Work out the finished part from the listing and answer in its coordinate system (mm). Give positions to 0.01 mm unless a question says otherwise; leave off trailing zeros. Write each loop counter-clockwise with the first axis right and the second up, starting at its lowest first coordinate (ties: lowest second). Pieces come first, ordered by that corner, then holes. Notation, with made-up numbers: (-3.75, 69) -> (50.25, 69) arc R34 ccw to (50.25, 102) -> close; hole circle Ø9 at (86.5, 26). An arc over 180 degrees is marked (long way). Use a Markdown table: item, result. Add a question column.
Q1. Section C-C, the plane x = -95.25 is taken. Give the vertices of the cut face in (y, z).
Q2. Section B-B, the plane y = 19.05 is taken. Give the vertices of the cut face in (x, z) (3 decimals), plus the area to 3 significant figures.
Q3. Each of these flat-tipped pins is pushed along its axis until it touches: pin 1 Ø3.5 at (x, z) = (82.55, 6.35) entering from -Y; pin 2 Ø9 at (x, y) = (84.78, 19.05) entering from +Z; pin 3 Ø3 at (x, z) = (0, 6.35) entering from -Y. Where does it stop, or does it pass through?
Q4. Consider line 1 (X direction, y = -63.5, z = 5.5); line 2 (Y direction, x = -95.25, z = 6.75); line 3 (X direction, y = -61.5, z = 2.5). Determine where each line is inside the solid, lowest interval first.
Q5. Section A-A, the plane y = -63.5 is taken. Give the vertices of the cut face in (x, z).
Q6. Section D-D, the plane y = -5 is taken. Give the vertices of the cut face in (x, z).
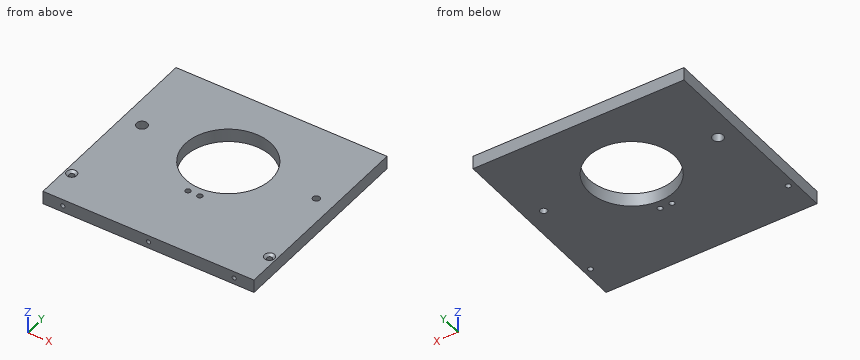
from build123d import *

# Parameters (mm, degrees)
SKETCH1_W                                          = 203.2
SKETCH1_H                                          = 190.5
BOSS_EXTRUDE1_DEPTH                                = 12.7
SKETCH2_R                                          = 41.275
SKETCH2_R_2                                        = 5.1435
SKETCH2_R_3                                        = 3.3655
CUT_EXTRUDE1_DEPTH                                 = 140.844243714
F_10_32_TAPPED_HOLE1_D                             = 4.0386
F_10_32_TAPPED_HOLE1_DEPTH                         = 25.4
F_10_32_TAPPED_HOLE1_TIP                           = 1.213317848
CSK_FOR_10_FLAT_HEAD_MACHINE_SCREW_100_D           = 4.9784
CSK_FOR_10_FLAT_HEAD_MACHINE_SCREW_100_CSINK_D     = 9.779
CSK_FOR_10_FLAT_HEAD_MACHINE_SCREW_100_CSINK_ANGLE = 100
F_7_0_201_DIAMETER_HOLE1_D                         = 5.1054


with BuildPart() as part:
    # Sketch1 → Boss-Extrude1 (new body)
    with BuildSketch(Plane.XY):
        Rectangle(SKETCH1_W, SKETCH1_H)
    extrude(amount=BOSS_EXTRUDE1_DEPTH)

    # Sketch2 → Cut-Extrude1 (cut, through all)
    with BuildSketch(Plane.XY.offset(12.7)):
        with Locations((0, 19.05)):
            Circle(SKETCH2_R)
        with Locations((-83.109250243, 19.05)):
            Circle(SKETCH2_R_2)
        with Locations((84.784749757, 19.05)):
            Circle(SKETCH2_R_3)
    extrude(amount=-CUT_EXTRUDE1_DEPTH, mode=Mode.SUBTRACT)

    # #10-32 Tapped Hole1
    with Locations(Plane(origin=(0, -95.25, 0), x_dir=(-1, 0, 0), z_dir=(0, -1, 0))):
        with Locations((82.55, -6.35), (0, -6.35), (-82.55, -6.35)):
            Hole(F_10_32_TAPPED_HOLE1_D / 2, depth=F_10_32_TAPPED_HOLE1_DEPTH)
            with Locations((0, 0, -(F_10_32_TAPPED_HOLE1_DEPTH + F_10_32_TAPPED_HOLE1_TIP / 2))):  # 118° drill point
                Cone(0, F_10_32_TAPPED_HOLE1_D / 2, F_10_32_TAPPED_HOLE1_TIP, mode=Mode.SUBTRACT)

    # CSK for #10 Flat Head Machine Screw (100)1 (through all)
    with Locations(Plane.XY.offset(12.7)):
        with Locations((-95.25, -63.5), (95.25, -63.5)):
            CounterSinkHole(CSK_FOR_10_FLAT_HEAD_MACHINE_SCREW_100_D / 2, CSK_FOR_10_FLAT_HEAD_MACHINE_SCREW_100_CSINK_D / 2, counter_sink_angle=CSK_FOR_10_FLAT_HEAD_MACHINE_SCREW_100_CSINK_ANGLE)

    # #7 (0.201) Diameter Hole1 (through all)
    with Locations(Plane.XY.offset(12.7)):
        with Locations((-5.715, -30.1625), (5.715, -30.1625)):
            Hole(F_7_0_201_DIAMETER_HOLE1_D / 2)


solid = part.part
Result set:
| question | item | result |
|---|---|---|
| 1 | outline | (-95.25, 0) -> (-65.99, 0) -> (-65.99, 10.69) -> (-68.39, 12.7) -> (-95.25, 12.7) -> close; (-61.01, 0) -> (95.25, 0) -> (95.25, 12.7) -> (-58.61, 12.7) -> (-61.01, 10.69) -> close |
| 2 | outline | (-101.6, 0) -> (-88.253, 0) -> (-88.253, 12.7) -> (-101.6, 12.7) -> close; (-77.966, 0) -> (-41.275, 0) -> (-41.275, 12.7) -> (-77.966, 12.7) -> close; (41.275, 0) -> (81.419, 0) -> (81.419, 12.7) -> (41.275, 12.7) -> close; (88.15, 0) -> (101.6, 0) -> (101.6, 12.7) -> (88.15, 12.7) -> close |
| 2 | area | 1,320 mm2 |
| 3 | pin 1 | stops at y = -69.69 |
| 3 | pin 2 | stops at z = 12.7 |
| 3 | pin 3 | stops at y = -69.54 |
| 4 | line 1 | x = -101.6 to -97.74, -92.76 to 92.76, 97.74 to 101.6 |
| 4 | line 2 | y = -95.25 to -65.99, -61.01 to 95.25 |
| 4 | line 3 | x = -101.6 to -96.73, -93.77 to 93.77, 96.73 to 101.6 |
| 5 | outline | (-101.6, 0) -> (-97.74, 0) -> (-97.74, 10.69) -> (-100.14, 12.7) -> (-101.6, 12.7) -> close; (-92.76, 0) -> (92.76, 0) -> (92.76, 10.69) -> (90.36, 12.7) -> (-90.36, 12.7) -> (-92.76, 10.69) -> close; (97.74, 0) -> (101.6, 0) -> (101.6, 12.7) -> (100.14, 12.7) -> (97.74, 10.69) -> close |
| 6 | outline | (-101.6, 0) -> (-33.54, 0) -> (-33.54, 12.7) -> (-101.6, 12.7) -> close; (33.54, 0) -> (101.6, 0) -> (101.6, 12.7) -> (33.54, 12.7) -> close |
